Can you work these out from the model? Positions are in its coordinate system, mm. Round coordinates to 2 decimals unless told otherwise and drop trailing zeros. Write each loop counter-clockwise with the first axis right and the second up, starting at its lowest first coordinate (ties: lowest second). Pieces come first, ordered by that corner, then holes. Notation, with made-up numbers: (12, 1) -> (52, 1) arc R28 ccw to (52, 40) -> close; hole circle Ø2 at (43, -40). An arc over 180 degrees is marked (long way). Write item = value, one per line. Start each with the question number.
1) Imagine slicing it at A-A, the plane y = 1.45. Please give me the cut outline in (x, z), then the cut area to 3 significant figures.
2) Imagine slicing it at B-B, the plane x = 0. Please give me the cut outline in (y, z).
3) If I drill on line 1 (Z direction, x = 0, y = 2.1); line 2 (Z direction, x = -140, y = 0.85), over which ranges is the centre line in solid material (lowest first)?
4) Imagine slicing it at C-C, the plane z = 0. Please give me the cut outline in (x, y).
5) I'm going to push flat-ended pins straight in: pin 1 (5 mm diameter, centred on x = 140, z = -140, fed in from +Y) (3 decimals); pin 2 (22.5 mm diameter, centred on x = 0, z = 71.75, fed in from -Y). Where does each tip first touch, or does it pass through?
from build123d import *

# Parameters (mm, degrees)
SKETCH1_W           = 300
SKETCH1_H           = 300
BOSS_EXTRUDE1_DEPTH = 4
CUT_EXTRUDE1_REACH  = 6
SKETCH2_R           = 3.25
CUT_EXTRUDE2_REACH  = 6
SKETCH3_R           = 20.5
CUT_EXTRUDE3_REACH  = 6
SKETCH4_R           = 7


with BuildPart() as part:
    # Sketch1 → Boss-Extrude1 (new body)
    with BuildSketch(Plane(origin=(0, 0, 0), x_dir=(1, 0, 0), z_dir=(0, 1, 0))):
        Rectangle(SKETCH1_W, SKETCH1_H)
    extrude(amount=BOSS_EXTRUDE1_DEPTH)

    # Sketch2 → Cut-Extrude1 (cut, up to next)
    with BuildSketch(Plane(origin=(0, 4, 0), x_dir=(1, 0, 0), z_dir=(0, 1, 0)), mode=Mode.PRIVATE) as cut_extrude1_sk1:
        with Locations((-140, 140)):
            Circle(SKETCH2_R)
    cut_extrude1_tool1 = extrude(cut_extrude1_sk1.sketch, amount=-CUT_EXTRUDE1_REACH, mode=Mode.PRIVATE) & part.part
    add(cut_extrude1_tool1.solids().sort_by_distance((-140, 4, -140))[0], mode=Mode.SUBTRACT)
    # Sketch2 → Cut-Extrude1 (cut, up to next)
    with BuildSketch(Plane(origin=(0, 4, 0), x_dir=(1, 0, 0), z_dir=(0, 1, 0)), mode=Mode.PRIVATE) as cut_extrude1_sk2:
        with Locations((140, 140)):
            Circle(SKETCH2_R)
    cut_extrude1_tool2 = extrude(cut_extrude1_sk2.sketch, amount=-CUT_EXTRUDE1_REACH, mode=Mode.PRIVATE) & part.part
    add(cut_extrude1_tool2.solids().sort_by_distance((140, 4, -140))[0], mode=Mode.SUBTRACT)
    # Sketch2 → Cut-Extrude1 (cut, up to next)
    with BuildSketch(Plane(origin=(0, 4, 0), x_dir=(1, 0, 0), z_dir=(0, 1, 0)), mode=Mode.PRIVATE) as cut_extrude1_sk3:
        with Locations((140, -140)):
            Circle(SKETCH2_R)
    cut_extrude1_tool3 = extrude(cut_extrude1_sk3.sketch, amount=-CUT_EXTRUDE1_REACH, mode=Mode.PRIVATE) & part.part
    add(cut_extrude1_tool3.solids().sort_by_distance((140, 4, 140))[0], mode=Mode.SUBTRACT)
    # Sketch2 → Cut-Extrude1 (cut, up to next)
    with BuildSketch(Plane(origin=(0, 4, 0), x_dir=(1, 0, 0), z_dir=(0, 1, 0)), mode=Mode.PRIVATE) as cut_extrude1_sk4:
        with Locations((-140, -140)):
            Circle(SKETCH2_R)
    cut_extrude1_tool4 = extrude(cut_extrude1_sk4.sketch, amount=-CUT_EXTRUDE1_REACH, mode=Mode.PRIVATE) & part.part
    add(cut_extrude1_tool4.solids().sort_by_distance((-140, 4, 140))[0], mode=Mode.SUBTRACT)

    # Sketch3 → Cut-Extrude2 (cut, up to next)
    with BuildSketch(Plane(origin=(0, 4, 0), x_dir=(1, 0, 0), z_dir=(0, 1, 0)), mode=Mode.PRIVATE) as cut_extrude2_sk1:
        Circle(SKETCH3_R)
    cut_extrude2_tool1 = extrude(cut_extrude2_sk1.sketch, amount=-CUT_EXTRUDE2_REACH, mode=Mode.PRIVATE) & part.part
    add(cut_extrude2_tool1.solids().sort_by_distance((0, 4, 0))[0], mode=Mode.SUBTRACT)

    # Sketch4 → Cut-Extrude3 (cut, up to next)
    with BuildSketch(Plane(origin=(0, 4, 0), x_dir=(1, 0, 0), z_dir=(0, 1, 0)), mode=Mode.PRIVATE) as cut_extrude3_sk1:
        with Locations((0, 71.75)):
            Circle(SKETCH4_R)
    cut_extrude3_tool1 = extrude(cut_extrude3_sk1.sketch, amount=-CUT_EXTRUDE3_REACH, mode=Mode.PRIVATE) & part.part
    add(cut_extrude3_tool1.solids().sort_by_distance((0, 4, -71.75))[0], mode=Mode.SUBTRACT)
    # Sketch4 → Cut-Extrude3 (cut, up to next)
    with BuildSketch(Plane(origin=(0, 4, 0), x_dir=(1, 0, 0), z_dir=(0, 1, 0)), mode=Mode.PRIVATE) as cut_extrude3_sk2:
        with Locations((0, -71.75)):
            Circle(SKETCH4_R)
    cut_extrude3_tool2 = extrude(cut_extrude3_sk2.sketch, amount=-CUT_EXTRUDE3_REACH, mode=Mode.PRIVATE) & part.part
    add(cut_extrude3_tool2.solids().sort_by_distance((0, 4, 71.75))[0], mode=Mode.SUBTRACT)


solid = part.part
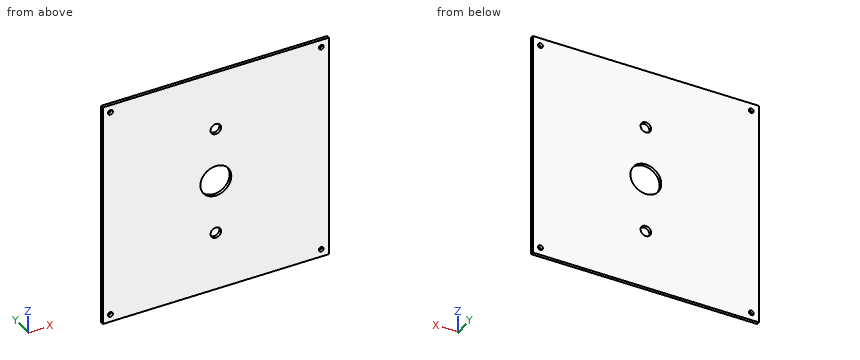
Reported:
q1.outline = (-150, -150) -> (150, -150) -> (150, 150) -> (-150, 150) -> close; hole circle Ø6.5 at (-140, -140); hole circle Ø6.5 at (-140, 140); hole circle Ø41 at (0, 0); hole circle Ø14 at (0, -71.75); hole circle Ø14 at (0, 71.75); hole circle Ø6.5 at (140, -140); hole circle Ø6.5 at (140, 140)
q1.area = 88,200 mm²
q2.outline = (0, -150) -> (4, -150) -> (4, -78.75) -> (0, -78.75) -> close; (0, -64.75) -> (4, -64.75) -> (4, -20.5) -> (0, -20.5) -> close; (0, 20.5) -> (4, 20.5) -> (4, 64.75) -> (0, 64.75) -> close; (0, 78.75) -> (4, 78.75) -> (4, 150) -> (0, 150) -> close
q3.line_1 = -150 to -78.75, -64.75 to -20.5, 20.5 to 64.75, 78.75 to 150
q3.line_2 = -150 to -143.25, -136.75 to 136.75, 143.25 to 150
q4.outline = (-150, 0) -> (-20.5, 0) -> (-20.5, 4) -> (-150, 4) -> close; (20.5, 0) -> (150, 0) -> (150, 4) -> (20.5, 4) -> close
q5.pin_1 = through
q5.pin_2 = 0
